Geometry check sheet. Reference: the model listing, model coordinates, mm. A direction names the side the tool comes from. Coordinates: 2 decimals unless noted, no trailing zeros. Loops run counter-clockwise (first coordinate to the right, second up) from the corner with the lowest first, then second, coordinate; pieces in that order, holes last. Notation, with made-up numbers: (1, -11) -> (26, -11) arc R19 ccw to (26, -1) -> close; hole circle Ø6 at (85.5, 59). An arc over 180 degrees is marked (long way). Answer as a JSON object with one key per item and string values.
from build123d import *

# Parameters (mm, degrees)
F0_W            = 195
F0_H            = 125
F0_W_2          = 175
F0_H_2          = 105
F1_DEPTH        = 35
F2_DEPTH        = 10
F3_W            = 40
F3_H            = 10
F3_W_2          = 10
F3_H_2          = 20
F4_DEPTH        = 20
F5_W            = 159
F5_H            = 89
F6_DEPTH        = 25
F8_W            = 30
F8_H            = 110
F9_DEPTH        = 10
F10_W           = 11
F10_H           = 11
F11_DEPTH       = 5
F12_DEPTH       = 5
F15_D           = 5
F15_DEPTH       = 12
F15_CBORE_D     = 10
F15_CBORE_DEPTH = 6
F15_TIP         = 1.5021515476
F16_D           = 5
F16_DEPTH       = 12
F16_CBORE_D     = 10
F16_CBORE_DEPTH = 6
F16_TIP         = 1.5021515476
F17_R           = 6
F18_R           = 6
F7_W            = 11
F7_H            = 11
F19_DEPTH       = 5


with BuildPart() as f1:
    # F0 (on Top) → F1 (new body)
    with BuildSketch(Plane.XY):
        Rectangle(F0_W, F0_H)
        Rectangle(F0_W_2, F0_H_2, mode=Mode.SUBTRACT)
    extrude(amount=F1_DEPTH)

    # F0 (on Top) → F2 (join)
    with BuildSketch(Plane.XY):
        Rectangle(F0_W_2, F0_H_2)
    extrude(amount=F2_DEPTH)

    # F3 (on face) → F4 (cut)
    with BuildSketch(Plane.XY.offset(35)):
        with Locations((0, 57.5)):
            Rectangle(F3_W, F3_H)
        with Locations((92.5, 37.5)):
            Rectangle(F3_W_2, F3_H_2)
    extrude(amount=-F4_DEPTH, mode=Mode.SUBTRACT)

    # F5 (on face) → F6 (cut)
    with BuildSketch(Plane.XY.offset(10)):
        Rectangle(F5_W, F5_H)
    extrude(amount=-F6_DEPTH, mode=Mode.SUBTRACT)

    # F8 (on Top) → F9 (join)
    with BuildSketch(Plane.XY):
        Rectangle(F8_W, F8_H)
    extrude(amount=F9_DEPTH)

    # F10 (on Top) → F11 (cut)
    with BuildSketch(Plane.XY):
        with Locations((0, 32.5)):
            Rectangle(F10_W, F10_H)
    extrude(amount=-F11_DEPTH, mode=Mode.SUBTRACT)

    # F10 (on Top) → F12 (cut)
    with BuildSketch(Plane.XY):
        with Locations((0, 32.5)):
            Rectangle(F10_W, F10_H)
    extrude(amount=F12_DEPTH, mode=Mode.SUBTRACT)

    # F15
    with Locations(Plane(origin=(-97.5, 0, 0), x_dir=(0, -1, 0), z_dir=(-1, 0, 0))):
        with Locations((-32.5, 25), (32.5, 25)):
            CounterBoreHole(F15_D / 2, F15_CBORE_D / 2, F15_CBORE_DEPTH, depth=F15_DEPTH)
            with Locations((0, 0, -(F15_DEPTH + F15_TIP / 2))):  # 118° drill point
                Cone(0, F15_D / 2, F15_TIP, mode=Mode.SUBTRACT)

    # F16
    with Locations(Plane(origin=(0, 62.5, 0), x_dir=(-1, 0, 0), z_dir=(0, 1, 0))):
        with Locations((-57.5, 25), (57.5, 25)):
            CounterBoreHole(F16_D / 2, F16_CBORE_D / 2, F16_CBORE_DEPTH, depth=F16_DEPTH)
            with Locations((0, 0, -(F16_DEPTH + F16_TIP / 2))):  # 118° drill point
                Cone(0, F16_D / 2, F16_TIP, mode=Mode.SUBTRACT)

    # F17
    f17_edges = [f1.edges().sort_by_distance(p)[0] for p in [
        (79.5, 0, 0),
        (47.25, 44.5, 0),
        (15, 0, 0),
        (47.25, -44.5, 0),
        (-15, 0, 0),
        (-47.25, 44.5, 0),
        (-79.5, 0, 0),
        (-47.25, -44.5, 0),
    ]]
    fillet(f17_edges, radius=F17_R)

    # F18
    f18_edges = [f1.edges().sort_by_distance(p)[0] for p in [
        (0, 62.5, 0),
        (97.5, 0, 0),
        (0, -62.5, 0),
        (-97.5, 0, 0),
        (-97.5, 62.5, 17.5),
        (97.5, 62.5, 17.5),
        (97.5, -62.5, 17.5),
        (-97.5, -62.5, 17.5),
    ]]
    fillet(f18_edges, radius=F18_R)

    # F7 (on face) → F19 (cut)
    with BuildSketch(Plane.XZ.offset(62.5)):
        with Locations((0, 17.5)):
            Rectangle(F7_W, F7_H)
    extrude(amount=-F19_DEPTH, mode=Mode.SUBTRACT)


solid = f1.part
1. Depth check by flat-ended pin: P1, Ø11, axis at x = 93.5, z = 29, coming from the +Y side; P2, Ø6, axis at y = -32.5, z = 25, coming from the -X side; P3, Ø3, axis at y = -32.5, z = 25, coming from the -X side; P4, Ø3, axis at x = 57, y = -47.5, coming from the +Z side. Enter the tip coordinate at first touch or a pass-through.
Evaluation:
{"P1": "stops at y = 62.5", "P2": "stops at x = -91.5", "P3": "stops at x = 87.5", "P4": "stops at z = 10"}
2. Section check B-B, the plane x = -57.5. Record the boundary of the cut face in (y, z), then the cut area to 3 significant figures.
Evaluation:
{"outline": "(-62.5, 6) arc R6 ccw to (-56.5, 0) -> (-50.5, 0) arc R6 ccw to (-44.5, 6) -> (-44.5, 10) -> (-52.5, 10) -> (-52.5, 35) -> (-62.5, 35) -> close; (44.5, 6) arc R6 ccw to (50.5, 0) -> (56.5, 0) arc R6 ccw to (62.5, 6) -> (62.5, 20) -> (56.5, 20) -> (56.5, 22.5) -> (52.5, 22.5) -> (52.5, 10) -> (44.5, 10) -> close; (52.5, 27.5) -> (56.5, 27.5) -> (56.5, 30) -> (62.5, 30) -> (62.5, 35) -> (52.5, 35) -> close", "area": "749 mm^2"}
3. Thickness scan on probe 1 along Y at (x, z) = (22.5, 32); probe 2 along X at (y, z) = (-44, 24); probe 3 along Z at (x, y) = (-57.5, 55.1). Record the ranges inside material, lowest first. Write a range as from..to.
Evaluation:
{"probe 1": "y = -62.5..-52.5, 52.5..62.5", "probe 2": "x = -97.5..-87.5, 87.5..97.5", "probe 3": "z = 0..22.5, 27.5..35"}
4. Section check C-C, the plane y = 32.5. State how many separate pieces and enclosed holes the cut face has, then the cut area to 3 significant figures.
Evaluation:
{"separate pieces": "4", "enclosed holes": "0", "area": "779 mm^2"}
5. Section check D-D, the plane x = -29.5. Record the boundary of the cut face in (y, z), then the cut area to 3 significant figures.
Evaluation:
{"outline": "(-62.5, 6) arc R6 ccw to (-56.5, 0) -> (-50.5, 0) arc R6 ccw to (-44.5, 6) -> (-44.5, 10) -> (-52.5, 10) -> (-52.5, 35) -> (-62.5, 35) -> close; (44.5, 6) arc R6 ccw to (50.5, 0) -> (56.5, 0) arc R6 ccw to (62.5, 6) -> (62.5, 35) -> (52.5, 35) -> (52.5, 10) -> (44.5, 10) -> close", "area": "829 mm^2"}
6. Mould release check, pull along Z, two halves, no side actions. Record for faces 1 (the face through (-46.714, 46.304, 1.711)), 2 (the face through (0, 38, 2)), 3 (the face through (-56.42, 59.54, 20.12)): released by +Z, released by -Z, zero draft, split by the parting line, or undercut.
Evaluation:
{"face 1": "released by -Z", "face 2": "zero draft", "face 3": "undercut"}
7. Tool access check on faces 4 (the face through (-15, -1, 8)), 5 (the face through (0, -57.5, 18)), 6 (the face through (20, 57, 25)), 7 (the face through (-94.5, 36.5, 22)), 8 (the face through (60, 56.5, 24)). Record the directions out of +Z, -Z, +X, -X, +Y, -Y that give a thin tool (end or side, any length) a straight path to the whole face; none if there is none.
Evaluation:
{"face 4": "+Z, -Z", "face 5": "-Y", "face 6": "+Z, +Y", "face 7": "-X", "face 8": "+Y"}
8. Section check A-A, the plane y = 9. Record the boundary of the cut face in (x, z), then the cut area to 3 significant figures.
Evaluation:
{"outline": "(-97.5, 6) arc R6 ccw to (-91.5, 0) -> (-85.5, 0) arc R6 ccw to (-79.5, 6) -> (-79.5, 10) -> (-87.5, 10) -> (-87.5, 35) -> (-97.5, 35) -> close; (-15, 6) arc R6 ccw to (-9, 0) -> (9, 0) arc R6 ccw to (15, 6) -> (15, 10) -> (-15, 10) -> close; (79.5, 6) arc R6 ccw to (85.5, 0) -> (91.5, 0) arc R6 ccw to (97.5, 6) -> (97.5, 35) -> (87.5, 35) -> (87.5, 10) -> (79.5, 10) -> close", "area": "1,110 mm^2"}
